from build123d import *

# Parameters (mm, degrees)
SKETCH_1_R      = 1.65
SKETCH_1_R_2    = 2.15
SKETCH_1_R_3    = 10
SKETCH_1_R_4    = 11.2
SKETCH_1_R_5    = 2.65
EXTRUDE_1_DEPTH = 10
EXTRUDE_2_DEPTH = 10
SKETCH_4_W      = 10
SKETCH_4_H      = 5
SKETCH_4_R      = 2.5
EXTRUDE_3_DEPTH = 10


with BuildPart() as part:
    # 草图1 → 凸台-拉伸1 (new body)
    with BuildSketch(Plane(origin=(0, 0, 0), x_dir=(1, 0, 0), z_dir=(0, 1, 0))):
        with BuildLine():
            Line((-27.5, 0), (-27.5, 272.5))
            Line((-27.5, 272.5), (27.5, 272.5))
            Line((27.5, 272.5), (27.5, 0))
            ThreePointArc((27.5, 0), (0, -27.5), (-27.5, 0))
        make_face()
        with Locations(Location((0, 10.25, 0), (0, 0, 270))):
            Circle(SKETCH_1_R, mode=Mode.SUBTRACT)
        with Locations(Location((8.876760389, 5.125, 0), (0, 0, 270))):
            Circle(SKETCH_1_R, mode=Mode.SUBTRACT)
        with Locations(Location((8.876760389, -5.125, 0), (0, 0, 270))):
            Circle(SKETCH_1_R, mode=Mode.SUBTRACT)
        with Locations(Location((0, -10.25, 0), (0, 0, 270))):
            Circle(SKETCH_1_R, mode=Mode.SUBTRACT)
        with Locations(Location((-8.876760389, -5.125, 0), (0, 0, 270))):
            Circle(SKETCH_1_R, mode=Mode.SUBTRACT)
        with Locations(Location((-8.876760389, 5.125, 0), (0, 0, 270))):
            Circle(SKETCH_1_R, mode=Mode.SUBTRACT)
        with Locations(Location((-17.67766953, 262.67766953, 0), (0, 0, 270))):
            Circle(SKETCH_1_R_2, mode=Mode.SUBTRACT)
        with Locations(Location((17.67766953, 262.67766953, 0), (0, 0, 270))):
            Circle(SKETCH_1_R_2, mode=Mode.SUBTRACT)
        with Locations(Location((17.67766953, 227.32233047, 0), (0, 0, 270))):
            Circle(SKETCH_1_R_2, mode=Mode.SUBTRACT)
        with Locations(Location((-17.67766953, 227.32233047, 0), (0, 0, 270))):
            Circle(SKETCH_1_R_2, mode=Mode.SUBTRACT)
        with Locations(Location((0, 245, 0), (0, 0, 270))):
            Circle(SKETCH_1_R_3, mode=Mode.SUBTRACT)
        with Locations(Location((-15.5, 85.5, 0), (0, 0, 270))):
            Circle(SKETCH_1_R, mode=Mode.SUBTRACT)
        with Locations(Location((15.5, 85.5, 0), (0, 0, 270))):
            Circle(SKETCH_1_R, mode=Mode.SUBTRACT)
        with Locations(Location((15.5, 54.5, 0), (0, 0, 270))):
            Circle(SKETCH_1_R, mode=Mode.SUBTRACT)
        with Locations(Location((-15.5, 54.5, 0), (0, 0, 270))):
            Circle(SKETCH_1_R, mode=Mode.SUBTRACT)
        with Locations(Location((0, 70, 0), (0, 0, 270))):
            Circle(SKETCH_1_R_4, mode=Mode.SUBTRACT)
        with Locations(Location((0, 35, 0), (0, 0, 270))):
            Circle(SKETCH_1_R_3, mode=Mode.SUBTRACT)
        with Locations(Location((-13.5, 157.5, 0), (0, 0, 270))):
            Circle(SKETCH_1_R_5, mode=Mode.SUBTRACT)
        with BuildLine():
            Line((-10, 105), (-10, 140))
            ThreePointArc((-10, 140), (0, 150), (10, 140))
            Line((10, 140), (10, 105))
            ThreePointArc((10, 105), (0, 95), (-10, 105))
        make_face(mode=Mode.SUBTRACT)
        with BuildLine():
            Line((-10, 175), (-10, 210))
            ThreePointArc((-10, 210), (0, 220), (10, 210))
            Line((10, 210), (10, 175))
            ThreePointArc((10, 175), (0, 165), (-10, 175))
        make_face(mode=Mode.SUBTRACT)
    extrude(amount=EXTRUDE_1_DEPTH)

    # 草图2 → 凸台-拉伸2 (add)
    with BuildSketch(Plane(origin=(0, 10, 0), x_dir=(1, 0, 0), z_dir=(0, 1, 0))):
        with BuildLine():
            Line((-27.5, 272.5), (-27.5, 0))
            ThreePointArc((-27.5, 0), (0, -27.5), (27.5, 0))
            Line((27.5, 0), (27.5, 272.5))
            Line((27.5, 272.5), (-27.5, 272.5))
        make_face()
        with BuildLine():
            ThreePointArc((-22.5, 0), (0, -22.5), (22.5, 0))
            Line((22.5, 0), (22.5, 222.5))
            Line((22.5, 222.5), (22.5, 267.5))
            Line((22.5, 267.5), (-22.5, 267.5))
            Line((-22.5, 267.5), (-22.5, 222.5))
            Line((-22.5, 222.5), (-22.5, 0))
        make_face(mode=Mode.SUBTRACT)
    extrude(amount=EXTRUDE_2_DEPTH)

    # 草图4 → 凸台-拉伸3 (add)
    # profile 1 of 8: a face of its own
    with BuildSketch(Plane(origin=(0, 10, 0), x_dir=(1, 0, 0), z_dir=(0, 1, 0))):
        with Locations((-17.5, 95)):
            Rectangle(SKETCH_4_W, SKETCH_4_H)
    # profile 2 of 8: a face of its own
    with BuildSketch(Plane(origin=(0, 10, 0), x_dir=(1, 0, 0), z_dir=(0, 1, 0))):
        with Locations((-17.5, 220)):
            Rectangle(SKETCH_4_W, SKETCH_4_H)
    # profile 3 of 8: a face of its own
    with BuildSketch(Plane(origin=(0, 10, 0), x_dir=(1, 0, 0), z_dir=(0, 1, 0))):
        with Locations((17.5, 220)):
            Rectangle(SKETCH_4_W, SKETCH_4_H)
    # profile 4 of 8: a face of its own
    with BuildSketch(Plane(origin=(0, 10, 0), x_dir=(1, 0, 0), z_dir=(0, 1, 0))):
        with Locations((17.5, 95)):
            Rectangle(SKETCH_4_W, SKETCH_4_H)
    # profile 5 of 8: a face of its own
    with BuildSketch(Plane(origin=(0, 10, 0), x_dir=(1, 0, 0), z_dir=(0, 1, 0))):
        with Locations((-17.5, 45)):
            Rectangle(SKETCH_4_W, SKETCH_4_H)
    # profile 6 of 8: a face of its own
    with BuildSketch(Plane(origin=(0, 10, 0), x_dir=(1, 0, 0), z_dir=(0, 1, 0))):
        with Locations((17.5, 45)):
            Rectangle(SKETCH_4_W, SKETCH_4_H)
    # profile 7 of 8: a face of its own
    with BuildSketch(Plane(origin=(0, 10, 0), x_dir=(1, 0, 0), z_dir=(0, 1, 0))):
        with BuildLine():
            Line((-22.5, 155), (-22.5, 160))
            Line((-22.5, 160), (-18.954356057, 160))
            ThreePointArc((-18.954356057, 160), (-7.5, 157.5), (-18.954356057, 155))
            Line((-18.954356057, 155), (-22.5, 155))
        make_face()
        with Locations(Location((-13.5, 157.5, 0), (0, 0, 90))):
            Circle(SKETCH_4_R, mode=Mode.SUBTRACT)
    # profile 8 of 8: a face of its own
    with BuildSketch(Plane(origin=(0, 10, 0), x_dir=(1, 0, 0), z_dir=(0, 1, 0))):
        with Locations((17.5, 157.5)):
            Rectangle(SKETCH_4_W, SKETCH_4_H)
    extrude(amount=EXTRUDE_3_DEPTH)


solid = part.part
Geometry check sheet. Reference: the model listing, model coordinates, mm. A direction names the side the tool comes from. Give positions to 0.01 mm unless a question says otherwise; leave off trailing zeros. Order: outer loops, then holes, each group sorted by start corner. A loop starts at its lowest first (then second) coordinate and runs counter-clockwise, first axis right, second up. Notation, with made-up numbers: (46, -2) - (95, -2) arc R6 cw to (95, 6) - close; hole circle Ø10 at (80, -17). An arc over 180 degrees is marked (long way). Use one line per item in the form item = value.
1) Sectioned sample at C-C (z = -214.5). Record the boundary of the cut face in (x, y).
Working result:
outline = (-27.5, 0) - (-8.93, 0) - (-8.93, 10) - (-22.5, 10) - (-22.5, 20) - (-27.5, 20) - close; (8.93, 0) - (27.5, 0) - (27.5, 20) - (22.5, 20) - (22.5, 10) - (8.93, 10) - close
2) Material ranges on probe 1 along X at (y, z) = (16.25, -243); probe 2 along X at (y, z) = (2.25, -10.25); probe 3 along Z at (x, y) = (-18.5, 18.25), recorded low to high. Write a range as from..to.
Working result:
probe_1 = -27.5..-22.5, 22.5..27.5
probe_2 = -27.5..-1.65, 1.65..27.5
probe_3 = -272.5..-267.5, -222.5..-217.5, -160.82..-154.18, -97.5..-92.5, -47.5..-42.5, 12.81..20.35
3) Sectioned sample at B-B (y = 7.5). Count the separate pieces of the cut face and the enclosed holes in it, and give its area (3 significant figures).
Working result:
separate_pieces = 1
enclosed_holes = 20
area = 13,000 mm^2
4) Draft check along Z on faces 1 (the face through (-27.5, 10, -138)), 2 (the face through (22.5, 15, -21)). Enter one of: released by +Z, released by -Z, zero draft, split by the parting line, or undercut.
Working result:
face_1 = zero draft
face_2 = undercut
5) Depth check by flat-ended pin: pin 1 Ø3 at (x, y) = (-21.5, 16.5) entering from +Z; pin 2 Ø3 at (x, z) = (-13.5, -12) entering from +Y; pin 3 Ø5 at (x, y) = (-18.5, 16) entering from +Z. Enter the tip coordinate at first touch or a pass-through.
Working result:
pin_1 = 18.87
pin_2 = 10
pin_3 = 22.37
6) Sectioned sample at A-A (z = -35). Record the boundary of the cut face in (x, y).
Working result:
outline = (-27.5, 0) - (-10, 0) - (-10, 10) - (-22.5, 10) - (-22.5, 20) - (-27.5, 20) - close; (10, 0) - (27.5, 0) - (27.5, 20) - (22.5, 20) - (22.5, 10) - (10, 10) - close
7) Access from +Z, -Z, +X, -X, +Y, -Y to the whole of each face (thin tool, end or side, straight path). Record for faces 3 (the face through (-10, 20, -157)), 4 (the face through (0, 5, -95)), 5 (the face through (12.5, 15, -95)).
Working result:
face_3 = +Z, -Z, +X, -X, +Y
face_4 = +Y, -Y
face_5 = +Y
